Source: three-view drawing plus pictorial views. Frame: mm from the lowest corner of the part. A direction names the side the tool comes from. Round coordinates to 2 decimals unless told otherwise and drop trailing zeros. Loops run counter-clockwise (first coordinate to the right, second up) from the corner with the lowest first, then second, coordinate; pieces in that order, holes last. Notation, with made-up numbers: (65.5, -35) -> (119.5, -35) arc R23 cw to (119.5, 1) -> close; hole circle Ø2 at (-19.5, 12.25). An arc over 180 degrees is marked (long way). Answer as a JSON object with one key per item and string values. Group by question number.
Item 1: Section query C-C on y = 4. Return loops of the section in (x, z).
Item 2: Section query D-D on z = 48.1. Return loops of the section in (x, y) (3 decimals), and give its area (4 significant figures).
Item 3: Section query A-A on y = 10. Return loops of the section in (x, z).
Item 4: Material intervals for line 1 (Z direction, x = 15, y = 13.9) (3 decimals); line 2 (Z direction, x = 6.5, y = 4.5); line 3 (Y direction, x = 5, z = 25.5), sorted ascending. Write a range as [from, to].
Item 5: Set-up query: the marked faces 4, 5 and 6. Return all of +Z, -Z, +X, -X, +Y, -Y with unobstructed straight access to the full face (end or side cutting, diameter ignored); none if empty.
Item 6: Draft query along Z for the marked faces 1, 2 and 3. Return one class per face: released by +Z, released by -Z, zero draft, split by the parting line, or undercut.
Item 7: Pin query (flat end, axial travel): pin 1 (0.9 mm diameter, centred on x = 9, y = 9, fed in from -Z); pin 2 (3.5 mm diameter, centred on x = 20.5, z = 44, fed in from -Y); pin 3 (6 mm diameter, centred on y = 5.5, z = 11.5, fed in from +X); pin 4 (8 mm diameter, centred on y = 5.5, z = 35, fed in from +X). Return the tip coordinate at first contact, or that it passes through.
Item 8: Section query B-B on x = 15. Return loops of the section in (y, z) (3 decimals), and give its area (3 significant figures).
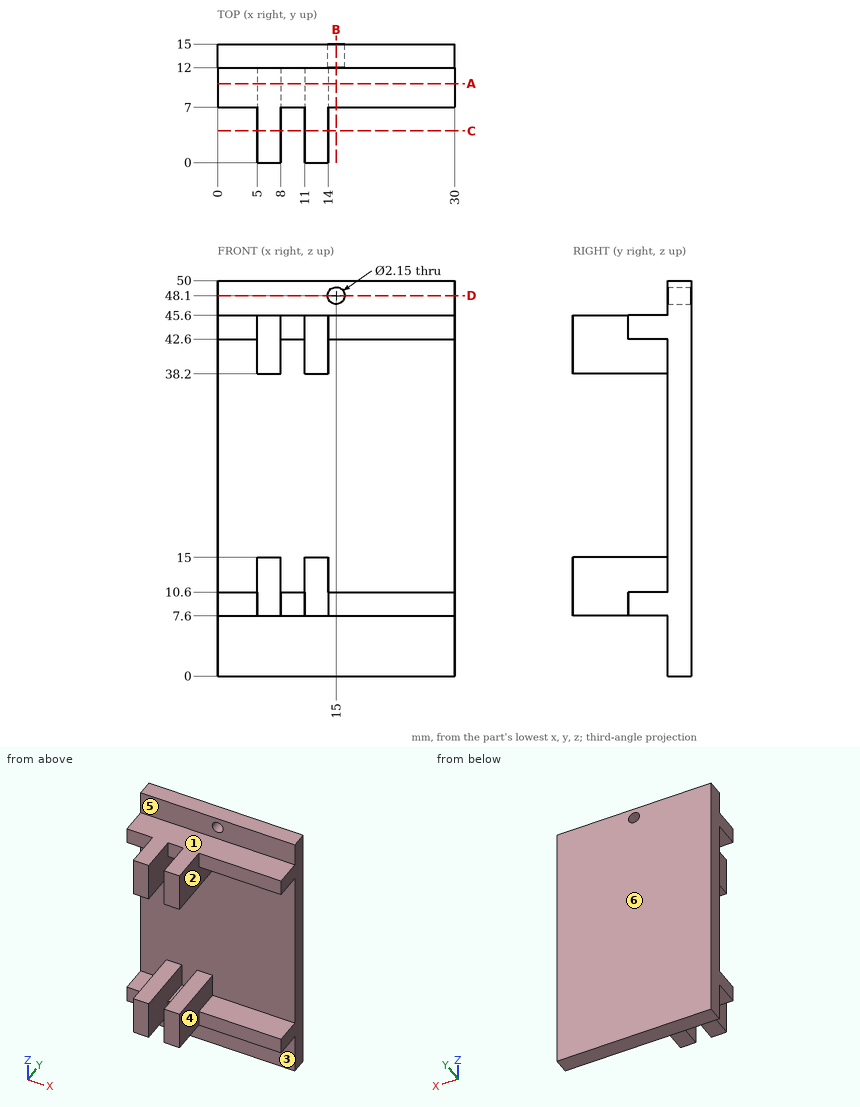
Solved:
{
 "1": {"outline": "(5, 7.6) -> (8, 7.6) -> (8, 15) -> (5, 15) -> close; (5, 38.2) -> (8, 38.2) -> (8, 45.6) -> (5, 45.6) -> close; (11, 7.6) -> (14, 7.6) -> (14, 15) -> (11, 15) -> close; (11, 38.2) -> (14, 38.2) -> (14, 45.6) -> (11, 45.6) -> close"},
 "2": {"outline": "(0, 12) -> (13.925, 12) -> (13.925, 15) -> (0, 15) -> close; (16.075, 12) -> (30, 12) -> (30, 15) -> (16.075, 15) -> close", "area": "83.55 mm²"},
 "3": {"outline": "(0, 7.6) -> (30, 7.6) -> (30, 10.6) -> (14, 10.6) -> (14, 15) -> (11, 15) -> (11, 10.6) -> (8, 10.6) -> (8, 15) -> (5, 15) -> (5, 10.6) -> (0, 10.6) -> close; (0, 42.6) -> (5, 42.6) -> (5, 38.2) -> (8, 38.2) -> (8, 42.6) -> (11, 42.6) -> (11, 38.2) -> (14, 38.2) -> (14, 42.6) -> (30, 42.6) -> (30, 45.6) -> (0, 45.6) -> close"},
 "4": {"line 1": "[0, 47.025], [49.175, 50]", "line 2": "[7.6, 15], [38.2, 45.6]", "line 3": "[12, 15]"},
 "5": {"face 4": "+X, -Y", "face 5": "+Z, +X, -X, -Y", "face 6": "+Z, -Z, +X, -X, +Y"},
 "6": {"face 1": "released by +Z", "face 2": "undercut", "face 3": "zero draft"},
 "7": {"pin 1": "z = 7.6", "pin 2": "y = 7", "pin 3": "x = 30", "pin 4": "x = 14"},
 "8": {"outline": "(7, 7.6) -> (12, 7.6) -> (12, 0) -> (15, 0) -> (15, 47.025) -> (12, 47.025) -> (12, 45.6) -> (7, 45.6) -> (7, 42.6) -> (12, 42.6) -> (12, 10.6) -> (7, 10.6) -> close; (12, 49.175) -> (15, 49.175) -> (15, 50) -> (12, 50) -> close", "area": "174 mm²"}
}
